Here's how the part is built. I have some questions about the finished solid (model axes, mm). Face numbers are marked on the shaded views. Round coordinates to 2 decimals unless told otherwise and drop trailing zeros. Write each loop counter-clockwise with the first axis right and the second up, starting at its lowest first coordinate (ties: lowest second). Pieces come first, ordered by that corner, then holes. Notation, with made-up numbers: (54, -22) -> (81, -22) arc R15 ccw to (81, 4) -> close; hole circle Ø2 at (28, -3.75). An arc over 180 degrees is marked (long way). Answer in a Markdown table with one row per item.
from build123d import *

# Parameters (mm, degrees)
SKETCH1_R           = 8
BOSS_EXTRUDE1_DEPTH = 2
CHAMFER1_SIZE       = 1
CHAMFER1_SIZE2      = 2.747477419
SKETCH2_R           = 2
CUT_EXTRUDE1_DEPTH  = 3


with BuildPart() as part:
    # Sketch1 → Boss-Extrude1 (new body)
    with BuildSketch(Plane(origin=(0, 0, 0), x_dir=(1, 0, 0), z_dir=(0, 1, 0))):
        Circle(SKETCH1_R)
    extrude(amount=BOSS_EXTRUDE1_DEPTH)

    # Chamfer1
    chamfer1_edges = [part.edges().sort_by_distance(p)[0] for p in [
        (-8, 2, 0),
    ]]
    chamfer1_side = [part.faces().sort_by_distance(p)[0] for p in [
        (-8, 1, 0),
    ]]
    chamfer(chamfer1_edges, length=CHAMFER1_SIZE, length2=CHAMFER1_SIZE2, reference=chamfer1_side[0])

    # Sketch2 → Cut-Extrude1 (cut, through all)
    with BuildSketch(Plane(origin=(0, 2, 0), x_dir=(1, 0, 0), z_dir=(0, 1, 0))):
        Circle(SKETCH2_R)
    extrude(amount=-CUT_EXTRUDE1_DEPTH, mode=Mode.SUBTRACT)


solid = part.part
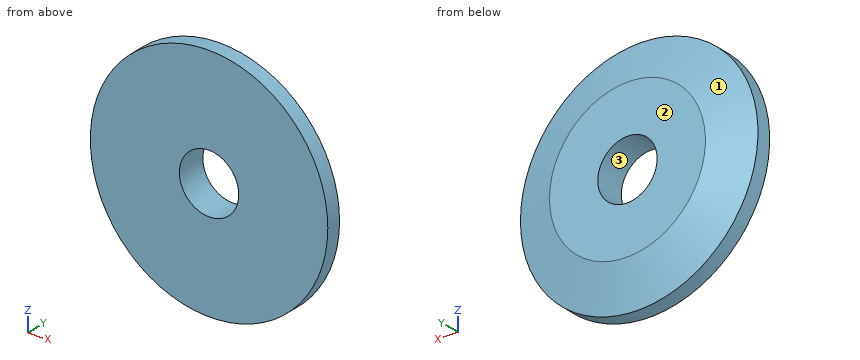
1) I want a section at A-A, the plane z = 0. List the corners of the cut face in (x, y) for me.
Response:
| item | result |
|---|---|
| outline | (-8, 0) -> (-2, 0) -> (-2, 2) -> (-5.25, 2) -> (-8, 1) -> close; (2, 0) -> (8, 0) -> (8, 1) -> (5.25, 2) -> (2, 2) -> close |
2) I want a section at B-B, the plane x = 0. List the corners of the cut face in (y, z) for me.
Response:
| item | result |
|---|---|
| outline | (0, -8) -> (1, -8) -> (2, -5.25) -> (2, -2) -> (0, -2) -> close; (0, 2) -> (2, 2) -> (2, 5.25) -> (1, 8) -> (0, 8) -> close |
3) I need wall thicknesses on line 1 (Z direction, x = 0, y = 0.7); line 2 (Z direction, x = -1.5, y = 0.8). Which ranges of each line are inside material? Lowest first, please. Write a range as [from, to].
Response:
| item | result |
|---|---|
| line 1 | z = [-8, -2], [2, 8] |
| line 2 | z = [-7.86, -1.32], [1.32, 7.86] |
4) We'd pull the mould along Z, two halves only. Please class the marked faces 1, 2 and 3: +Z half, -Z half, draft (parallel to the pull), parting line (faces both ways), or undercut.
Response:
| item | result |
|---|---|
| face 1 | parting line |
| face 2 | draft |
| face 3 | undercut |
5) I want a section at C-C, the plane y = 0.7. List the corners of the cut face in (x, z) for me, and give its area (3 significant figures).
Response:
| item | result |
|---|---|
| outline | circle Ø16 at (0, 0); hole circle Ø4 at (0, 0) |
| area | 188 mm^2 |
